Source: CAD feature listing. Evaluate the final solid. Frame: model axes, mm. A direction names the side the tool comes from. Round coordinates to 2 decimals unless told otherwise and drop trailing zeros. Write each loop counter-clockwise with the first axis right and the second up, starting at its lowest first coordinate (ties: lowest second). Pieces come first, ordered by that corner, then holes. Notation, with made-up numbers: (-13, 23) - (3, 23) arc R20 cw to (3, 32) - close; hole circle Ø7 at (-21.75, -30). An arc over 180 degrees is marked (long way). Write item = value, one per line. Start each with the question number.
Autodesk Inventor part; units mm, degrees
ref_plane "YZ Plane" through (0, 0, 0) normal (1, 0, 0) x (0, 1, 0)
ref_plane "XZ Plane" through (0, 0, 0) normal (0, 1, 0) x (-1, 0, 0)
ref_plane "XY Plane" through (0, 0, 0) normal (0, 0, 1) x (1, 0, 0)
sketch "Sketch1" plane through (0, 0, 0) normal (0, 0, 1) x (1, 0, 0)
  line L0 (0, 0) -> (50, 0)
  line L1 (50, 0) -> (50, 10)
  line L2 (50, 10) -> (0, 10)
  line L3 (0, 10) -> (0, 0)
  dimension "d0" = 50
  dimension "d1" = 10
extrude "Extrusion1" add sketch "Sketch1" along normal blind 6
sketch "Sketch2" plane through (0, 0, 0) normal (-1, 0, 0) x (0, 0, 1)
  circle A0 centre (6, 5) radius 3.5
  line L0 (6, 10) -> (6, 0)
  point P0 (0, 0)
  dimension "d4" = 7
extrude "Extrusion2" cut sketch "Sketch2" against normal through all
sketch "Sketch3" plane through (0, 0, 0) normal (0, 0, -1) x (-1, 0, 0)
  line L0 (-50, 0) -> (-50, 10)
  line L1 (0, 10) -> (0, 0)
  line L2 (-50, 10) -> (-38, 10)
  line L3 (-38, 10) -> (-38, 16)
  line L4 (-38, 16) -> (-50, 16)
  line L5 (-50, 16) -> (-50, 10)
  line L6 (0, 10) -> (-12, 10)
  line L7 (-12, 10) -> (-12, 16)
  line L8 (-12, 16) -> (0, 16)
  line L9 (0, 16) -> (0, 10)
  line L10 (0, 0) -> (-12, 0)
  line L11 (-12, 0) -> (-12, -6)
  line L12 (-12, -6) -> (0, -6)
  line L13 (0, -6) -> (0, 0)
  line L14 (-50, 0) -> (-38, 0)
  line L15 (-38, 0) -> (-38, -6)
  line L16 (-38, -6) -> (-50, -6)
  line L17 (-50, -6) -> (-50, 0)
  circle A0 centre (-44, 13) radius 1.5
  circle A1 centre (-6, 13) radius 1.5
  circle A2 centre (-6, -3) radius 1.5
  circle A3 centre (-44, -3) radius 1.5
  point P0 (-38, 13)
  point P1 (-12, 13)
  point P2 (-12, -3)
  point P3 (-50, -3)
  point P4 (-44, 16)
  point P5 (-6, 16)
  point P6 (-6, 0)
  point P7 (-44, 0)
  dimension "d15" = 12
  dimension "d16" = 6
  dimension "d17" = 12
  dimension "d18" = 6
  dimension "d19" = 12
  dimension "d20" = 6
  dimension "d21" = 12
  dimension "d22" = 6
  dimension "d23" = 3
  dimension "d24" = 3
  dimension "d25" = 3
  dimension "d26" = 3
extrude "Extrusion3" add sketch "Sketch3" against normal blind 3
sketch "Sketch4" plane through (0, 0, 6) normal (0, 0, 1) x (1, 0, 0)
  line L0 (50, 10) -> (0, 10)
  line L1 (0, 0) -> (50, 0)
  line L2 (15, 10) -> (35, 10)
  line L3 (35, 10) -> (35, 0)
  line L4 (35, 0) -> (15, 0)
  line L5 (15, 0) -> (15, 10)
  point P0 (25, 10)
  dimension "d29" = 20
extrude "Extrusion4" cut sketch "Sketch4" against normal blind 5
equation "\"d15\" = d21"
equation "\"d17\" = d21"
equation "\"d19\" = d21"
properties part number "bearing bed"
(1) Section C-C (x = 44). Return the cut outline in (y, z).
(2) Ray query, L1, parallel to Y at x = 44, z = 2.25; L2, parallel to X at y = 4.5, z = 2.4; L3, parallel to X at y = -2.25, z = 1.3. Return the intervals inside material, ascending. Write a range as from..to.
(3) Section B-B (z = 1.75). Return the cut outline in (x, y), plus the area to 3 significant figures.
(4) Section A-A (y = -3). Return the cut outline in (x, z).
(5) Reachability of faces 4 (the flat face through (7.4, -1.6, 3)), 5 (the flat face through (12, -3, 1)), 6 (the flat face through (12, 13, 1)) from +Z, -Z, +X, -X, +Y, -Y: full face, straight path, thin tool, end or side. Return the list, or none.
(6) Contact query for flat-ended pins moving along their axis: P1, Ø3, axis at x = 34, z = 3, coming from the -Y side; P2, Ø6.5, axis at x = 5.5, y = 13.5, coming from the +Z side; P3, Ø1, axis at x = 5.5, y = 3, coming from the +Z side. Output: stop coordinate, or through.
(7) Pull-direction query (Y, two-part tool) for faces 1 (the flat face through (42, 1, 6)), 2 (the cylindrical face through (7.4, 5.1, 2.5)), 3 (the flat face through (44, -6, 1)); classes: +Y half, -Y half, draft (parallel to the pull), parting line (faces both ways), or undercut.
(8) Section D-D (z = 5.2). Return the cut outline in (x, y), plus the area to 3 significant figures.
Solution:
q1.outline = (-6, 0) - (-4.5, 0) - (-4.5, 3) - (-6, 3) - close; (-1.5, 0) - (11.5, 0) - (11.5, 3) - (10, 3) - (10, 6) - (8.5, 6) arc R3.5 cw to (1.5, 6) - (0, 6) - (0, 3) - (-1.5, 3) - close; (14.5, 0) - (16, 0) - (16, 3) - (14.5, 3) - close
q2.L1 = -6..-4.5, -1.5..11.5, 14.5..16
q2.L2 = 0..15, 35..50
q2.L3 = 0..4.7, 7.3..12, 38..42.7, 45.3..50
q3.outline = (0, -6) - (12, -6) - (12, 0) - (15, 0) - (15, 10) - (12, 10) - (12, 16) - (0, 16) - close; (35, 0) - (38, 0) - (38, -6) - (50, -6) - (50, 16) - (38, 16) - (38, 10) - (35, 10) - close; hole circle Ø3 at (6, -3); hole circle Ø3 at (6, 13); hole circle Ø3 at (44, -3); hole circle Ø3 at (44, 13)
q3.area = 560 mm^2
q4.outline = (0, 0) - (4.5, 0) - (4.5, 3) - (0, 3) - close; (7.5, 0) - (12, 0) - (12, 3) - (7.5, 3) - close; (38, 0) - (42.5, 0) - (42.5, 3) - (38, 3) - close; (45.5, 0) - (50, 0) - (50, 3) - (45.5, 3) - close
q5.face_4 = +Z, +X, -X, -Y
q5.face_5 = +Z, -Z, -Y
q5.face_6 = +Z, -Z, +Y
q6.P1 = 0
q6.P2 = 3
q6.P3 = 3.55
q7.face_1 = draft
q7.face_2 = undercut
q7.face_3 = -Y half
q8.outline = (0, 0) - (15, 0) - (15, 1.59) - (0, 1.59) - close; (0, 8.41) - (15, 8.41) - (15, 10) - (0, 10) - close; (35, 0) - (50, 0) - (50, 1.59) - (35, 1.59) - close; (35, 8.41) - (50, 8.41) - (50, 10) - (35, 10) - close
q8.area = 95.6 mm^2
